Work out the finished part from the listing and answer in its coordinate system (mm). Coordinates: 2 decimals unless noted, no trailing zeros. Loops run counter-clockwise (first coordinate to the right, second up) from the corner with the lowest first, then second, coordinate; pieces in that order, holes last. Notation, with made-up numbers: (80.25, 0.5) -> (102.25, 0.5) arc R16 ccw to (102.25, 27.5) -> close; hole circle Ø8 at (-16.75, -30.75). An arc over 180 degrees is marked (long way). Use a Markdown table: item, result. Add a question column.
```python
from build123d import *

# Parameters (mm, degrees)
BOSS_EXTRUDE1_DEPTH  = 1.6
M3_CLEARANCE_HOLE1_D = 3.4


with BuildPart() as part:
    # Sketch1 → Boss-Extrude1 (new body)
    with BuildSketch(Plane(origin=(0, 0, 0), x_dir=(1, 0, 0), z_dir=(0, 1, 0))):
        with BuildLine():
            ThreePointArc((-65, 33.226495452), (-73, 0), (-65, -33.226495452))
            ThreePointArc((-65, -33.226495452), (-51.618795027, -51.618795027), (-33.226495452, -65))
            ThreePointArc((-33.226495452, -65), (0, -73), (33.226495452, -65))
            ThreePointArc((33.226495452, -65), (51.618795027, -51.618795027), (65, -33.226495452))
            ThreePointArc((65, -33.226495452), (70.971825396, -17.088007491), (73, 0))
            ThreePointArc((73, 0), (70.971825396, 17.088007491), (65, 33.226495452))
            ThreePointArc((65, 33.226495452), (51.618795027, 51.618795027), (33.226495452, 65))
            ThreePointArc((33.226495452, 65), (0, 73), (-33.226495452, 65))
            ThreePointArc((-33.226495452, 65), (-51.618795027, 51.618795027), (-65, 33.226495452))
        make_face()
    extrude(amount=BOSS_EXTRUDE1_DEPTH)

    # M3 Clearance Hole1 (through all)
    with Locations(Plane(origin=(0, 1.6, 0), x_dir=(1, 0, 0), z_dir=(0, 1, 0))):
        with Locations((0, 55), (55, 0), (-55, 0), (0, -55)):
            Hole(M3_CLEARANCE_HOLE1_D / 2)


solid = part.part
```
Item 1: Section C-C (y = 0.25) is taken. Determine the outline of the cut face in (x, z).
Item 2: Section A-A (x = 0) is taken. Determine the outline of the cut face in (y, z).
Item 3: Section B-B (z = -55) is taken. Determine the outline of the cut face in (x, y), then the cut area to 3 significant figures.
Item 4: Section D-D (z = 15) is taken. Determine the outline of the cut face in (x, y), then the cut area to 3 significant figures.
Item 5: Given pin 1 (2.5 mm diameter, centred on x = -55, z = 0, fed in from -Y), flat-ended and moving along its own axis, determine where the tip first touches the part or whether it passes through.
Item 6: For a pull along X with two mould halves and no side action, classify faces 1 (the face through (56.7, 0.79, -0.07)), 2 (the face through (-1, 1.6, -1)) as +X half, -X half, draft (parallel to the pull), parting line (faces both ways), or undercut.
Item 7: Find the intervals of material crossed by probe 1 along Z at (x, y) = (0.5, 0.45); probe 2 along X at (y, z) = (1.4, -54); probe 3 along X at (y, z) = (0.4, 54.5), in increasing order.
Output:
| question | item | result |
|---|---|---|
| 1 | outline | circle Ø146 at (0, 0); hole circle Ø3.4 at (-55, 0); hole circle Ø3.4 at (0, -55); hole circle Ø3.4 at (0, 55); hole circle Ø3.4 at (55, 0) |
| 2 | outline | (0, -73) -> (1.6, -73) -> (1.6, -56.7) -> (0, -56.7) -> close; (0, -53.3) -> (1.6, -53.3) -> (1.6, 53.3) -> (0, 53.3) -> close; (0, 56.7) -> (1.6, 56.7) -> (1.6, 73) -> (0, 73) -> close |
| 3 | outline | (-48, 0) -> (-1.7, 0) -> (-1.7, 1.6) -> (-48, 1.6) -> close; (1.7, 0) -> (48, 0) -> (48, 1.6) -> (1.7, 1.6) -> close |
| 3 | area | 148 mm2 |
| 4 | outline | (-71.44, 0) -> (71.44, 0) -> (71.44, 1.6) -> (-71.44, 1.6) -> close |
| 4 | area | 229 mm2 |
| 5 | pin 1 | passes through |
| 6 | face 1 | undercut |
| 6 | face 2 | draft |
| 7 | probe 1 | z = -73 to -56.62, -53.38 to 53.38, 56.62 to 73 |
| 7 | probe 2 | x = -49.12 to -1.37, 1.37 to 49.12 |
| 7 | probe 3 | x = -48.57 to -1.62, 1.62 to 48.57 |
